Design review of the part built by this model. Coordinates are the model's own, in mm. Coordinates: 2 decimals unless noted, no trailing zeros. Write each loop counter-clockwise with the first axis right and the second up, starting at its lowest first coordinate (ties: lowest second). Pieces come first, ordered by that corner, then holes. Notation, with made-up numbers: (25.5, -37.5) -> (62.5, -37.5) arc R32 ccw to (62.5, -9.5) -> close; hole circle Ø3 at (84.5, -24.5). An arc over 180 degrees is marked (long way). Answer in a Markdown table with one row per item. Add a question column.
Item 1: Take a section at A-A, the plane x = 21. Write out the cut boundary in (y, z), and give its area (3 significant figures).
Item 2: To check wall thickness, follow line 1 (Z direction, x = -2, y = 2.9); line 2 (X direction, y = 2.4, z = 0); line 3 (Z direction, x = 18, y = 0.8). State the ranges of each line that lie inside material, in increasing order.
Item 3: Take a section at D-D, the plane x = 10. Write out the cut boundary in (y, z).
Item 4: Draft analysis for pull direction X (two halves, no side actions). For faces 1 (the face through (17.74, 1.97, 1.18)), 2 (the face through (6, 0, -5)), 3 (the face through (28.347, 1.972, 3.366)), state which applies: released by +X, released by -X, zero draft, split by the parting line, or undercut.
Item 5: Take a section at B-B, the plane z = 0. Write out the cut boundary in (x, y), and give its area (3 significant figures).
Item 6: Take a section at C-C, the plane z = -4. Write out the cut boundary in (x, y).
from build123d import *

# Parameters (mm, degrees)
SKETCH1_R           = 2.55
BOSS_EXTRUDE1_DEPTH = 4
FILLET1_R           = 4
CUT_EXTRUDE1_DEPTH  = 4


with BuildPart() as part:
    # Sketch1 → Boss-Extrude1 (new body)
    with BuildSketch(Plane(origin=(0, 0, 0), x_dir=(1, 0, 0), z_dir=(0, 1, 0))):
        with BuildLine():
            Line((-9, 18), (-9, -9))
            Line((-9, -9), (20, -9))
            ThreePointArc((20, -9), (28.402583705, -3.224373905), (26.020682585, 6.689647316))
            Line((26.020682585, 6.689647316), (6.020682585, 24.689647316))
            ThreePointArc((6.020682585, 24.689647316), (-3.661547264, 26.22150057), (-9, 18))
        make_face()
        with Locations(Location((20, 0, 0), (0, 0, 270))):
            Circle(SKETCH1_R, mode=Mode.SUBTRACT)
        with Locations(Location((0, 18, 0), (0, 0, 270))):
            Circle(SKETCH1_R, mode=Mode.SUBTRACT)
    extrude(amount=BOSS_EXTRUDE1_DEPTH)

    # Fillet1
    fillet1_edges = [part.edges().sort_by_distance(p)[0] for p in [
        (-9, 2, 9),
    ]]
    fillet(fillet1_edges, radius=FILLET1_R)

    # Sketch2 → Cut-Extrude1 (cut)
    with BuildSketch(Plane.XZ):
        with BuildLine():
            ThreePointArc((-1.035786438, 3.585786438), (-1.782664146, 5.38890873), (-3.585786438, 6.135786438))
            Line((-3.585786438, 6.135786438), (-3.585786438, 3.585786438))
            Line((-3.585786438, 3.585786438), (-6.135786438, 3.585786438))
            ThreePointArc((-6.135786438, 3.585786438), (-3.585786438, 1.035786438), (-1.035786438, 3.585786438))
        make_face()
        with BuildLine():
            Line((-3.585786438, 3.585786438), (-3.585786438, 6.135786438))
            ThreePointArc((-3.585786438, 6.135786438), (-5.38890873, 5.38890873), (-6.135786438, 3.585786438))
            Line((-6.135786438, 3.585786438), (-3.585786438, 3.585786438))
        make_face()
    extrude(amount=-CUT_EXTRUDE1_DEPTH, mode=Mode.SUBTRACT)


solid = part.part
Answers:
| question | item | result |
|---|---|---|
| 1 | outline | (0, -11.21) -> (4, -11.21) -> (4, -2.35) -> (0, -2.35) -> close; (0, 2.35) -> (4, 2.35) -> (4, 8.94) -> (0, 8.94) -> close |
| 1 | area | 61.8 mm^2 |
| 2 | line 1 | z = -26.77 to -19.58, -16.42 to 1.59, 5.58 to 9 |
| 2 | line 2 | x = -9 to 17.45, 22.55 to 29 |
| 2 | line 3 | z = -13.91 to -1.58, 1.58 to 9 |
| 3 | outline | (0, -21.11) -> (4, -21.11) -> (4, 9) -> (0, 9) -> close |
| 4 | face 1 | undercut |
| 4 | face 2 | zero draft |
| 4 | face 3 | released by +X |
| 5 | outline | (-9, 0) -> (17.45, 0) -> (17.45, 4) -> (-9, 4) -> close; (22.55, 0) -> (29, 0) -> (29, 4) -> (22.55, 4) -> close |
| 5 | area | 132 mm^2 |
| 6 | outline | (-9, 0) -> (28.06, 0) -> (28.06, 4) -> (-9, 4) -> close |
